Could you check a few things on this model? Use its own coordinates, in mm. A direction names the side the tool comes from. Round coordinates to 2 decimals unless told otherwise and drop trailing zeros. Write each loop counter-clockwise with the first axis right and the second up, starting at its lowest first coordinate (ties: lowest second). Pieces come first, ordered by that corner, then holes. Notation, with made-up numbers: M -26,83 L -9,83 A23 ccw -9,91 Z; hole C 29,-23.75 d5. An arc over 180 degrees is marked long. One line per item, written item: value. Start each with the question number.
(1) I want a section at B-B on z = 1.5. Please give me the cut outline in (x, y), and give its area (3 significant figures).
(2) If I drill on L1, parallel to X at y = 7, z = 2.4; L2, parallel to X at y = 6.5, z = 3.85; L3, parallel to Y at x = -13.5, z = 3.3, over which ranges is the centre line in solid material (lowest first)?
(3) I want a section at A-A on x = 0. Please give me the cut outline in (y, z).
(4) Which directions (+Z, -Z, +X, -X, +Y, -Y) give clear straight access to the entire face, cutting with the end or side of a thin tool? Please do faces 1 (the face through (-19.7, 4.35, 2.46)), 2 (the face through (-44.52, -20.34, 2.46)).
(5) Thinking about a two-plate mould opening in X: for faces 3 (the face through (44.587, -17.987, 2.465)), 4 (the face through (-20.705, -13.945, 2.465)), 5 (the face through (52.396, -9.823, 2.465)), 6 (the face through (-1, -12, 5)), which applies, released by +X, released by -X, zero draft, split by the parting line, or undercut?
(6) I want a section at C-C on y = 8.5. Please give me the cut outline in (x, z), and give its area (3 significant figures).
(7) I want a section at D-D on x = -15.5. Please give me the cut outline in (y, z), and give its area (3 significant figures).
```python
from build123d import *

# Parameters (mm, degrees)
SKETCH1_R           = 11.5
BOSS_EXTRUDE1_DEPTH = 5


with BuildPart() as part:
    # Sketch1 → Boss-Extrude1 (new body)
    with BuildSketch(Plane.XY):
        with BuildLine():
            Line((30.863510665, -14.051466451), (58.700669217, -22.033643218))
            ThreePointArc((58.700669217, -22.033643218), (64.885164476, -18.605521518), (61.457042775, -12.421026259))
            Line((61.457042775, -12.421026259), (43.077002388, -7.150634488))
            ThreePointArc((43.077002388, -7.150634488), (20.295215387, 3.815450095), (2.451915541, 21.728615104))
            ThreePointArc((2.451915541, 21.728615104), (0, 23), (-2.451915541, 21.728615104))
            ThreePointArc((-2.451915541, 21.728615104), (-19.987359953, 4.143898292), (-42.303764549, -6.750694953))
            Line((-42.303764549, -6.750694953), (-61.457042775, -12.421026259))
            ThreePointArc((-61.457042775, -12.421026259), (-65.934476702, -20.948431695), (-57.240992184, -25.094198809))
            Line((-57.240992184, -25.094198809), (-31.431292557, -15.44876451))
            ThreePointArc((-31.431292557, -15.44876451), (-20.55006109, -13.957749538), (-10.079833017, -17.274170497))
            ThreePointArc((-10.079833017, -17.274170497), (0.33600307, -19.997177349), (10.654478564, -16.925781711))
            ThreePointArc((10.654478564, -16.925781711), (20.452273896, -13.332100428), (30.863510665, -14.051466451))
        make_face()
        Circle(SKETCH1_R, mode=Mode.SUBTRACT)
    extrude(amount=BOSS_EXTRUDE1_DEPTH)


solid = part.part
```
Found:
1. outline: M -61.46,-12.42 A6.68 ccw long -57.24,-25.09 L -31.43,-15.45 A25 cw -10.08,-17.27 A20 ccw 10.65,-16.93 A25 cw 30.86,-14.05 L 58.7,-22.03 A5 ccw 61.46,-12.42 L 43.08,-7.15 A75 cw 2.45,21.73 A3 ccw -2.45,21.73 A75 cw -42.3,-6.75 Z; hole C 0,0 d23
1. area: 1,910 mm²
2. L1: x = -16.24 to -9.12, 9.12 to 16.13
2. L2: x = -16.87 to -9.49, 9.49 to 16.75
2. L3: y = -15.61 to 9.35
3. outline: M -20,0 L -11.5,0 L -11.5,5 L -20,5 Z; M 11.5,0 L 23,0 L 23,5 L 11.5,5 Z
4. face 1: +Z, -Z, -X, +Y
4. face 2: +Z, -Z, -Y
5. face 3: undercut
5. face 4: undercut
5. face 5: released by +X
5. face 6: zero draft
6. outline: M -14.46,0 L -7.75,0 L -7.75,5 L -14.46,5 Z; M 7.75,0 L 14.36,0 L 14.36,5 L 7.75,5 Z
6. area: 66.7 mm²
7. outline: M -14.92,0 L 7.61,0 L 7.61,5 L -14.92,5 Z
7. area: 113 mm²
